Part print with two shaded views. Sizes in mm from the minimum x, y, z corner. Round coordinates to 2 decimals unless told otherwise and drop trailing zeros. Loops run counter-clockwise (first coordinate to the right, second up) from the corner with the lowest first, then second, coordinate; pieces in that order, holes last. Notation, with made-up numbers: (-13, 2) - (28, 2) arc R14 cw to (28, 26) - close; hole circle Ø5 at (42, -1.75). An arc over 180 degrees is marked (long way). One line per question, with ' | ' between items.
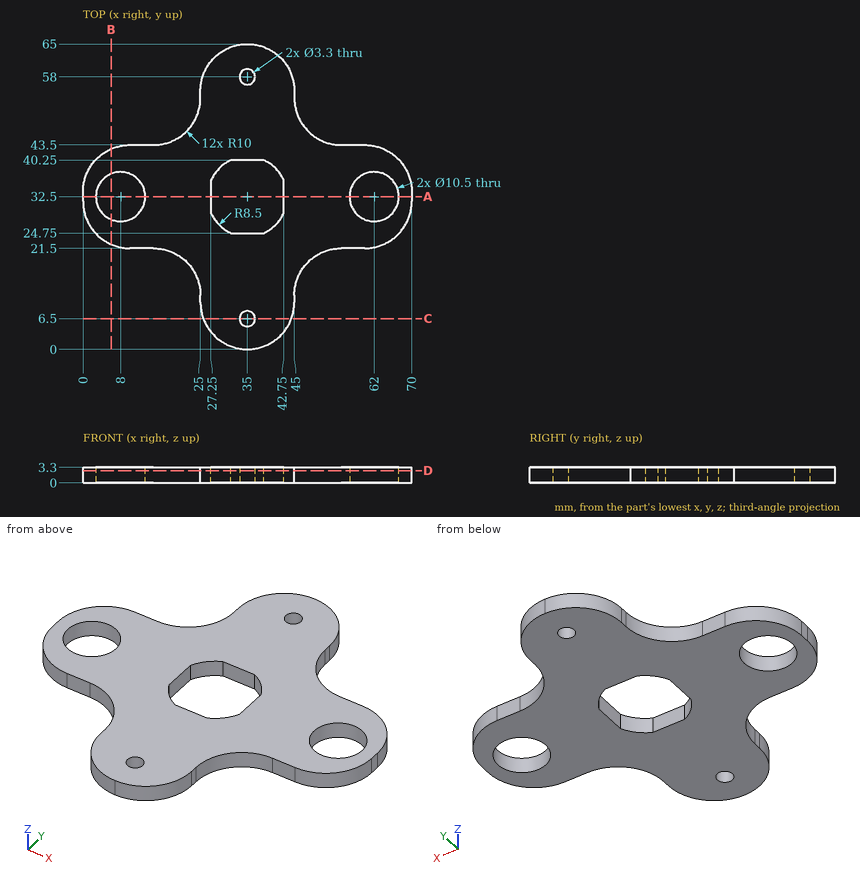
(1) Cut at C-C, the plane y = 6.5. Write the cut outline in (x, z), then the cut area to 3 significant figures.
Results found:
outline: (25.63, 0) - (33.35, 0) - (33.35, 3.3) - (25.63, 3.3) - close; (36.65, 0) - (44.37, 0) - (44.37, 3.3) - (36.65, 3.3) - close | area: 50.9 mm²
(2) Drop flat-ended pins along their axis: P1, Ø0.5, axis at y = 11, z = 1, coming from the +X side; P2, Ø1.7, axis at y = 10.5, z = 1.5, coming from the -X side; P3, Ø1.6, axis at x = 12.5, z = 2, coming from the +Y side. Give the stop position or say it passes through.
Results found:
P1: stops at x = 45 | P2: stops at x = 25 | P3: stops at y = 43.5
(3) Cut at B-B, the plane x = 6. Write the cut outline in (y, z) (3 decimals).
Results found:
outline: (22.335, 0) - (27.646, 0) - (27.646, 3.3) - (22.335, 3.3) - close; (37.354, 0) - (42.665, 0) - (42.665, 3.3) - (37.354, 3.3) - close
(4) Cut at D-D, the plane z = 2.6. State how many separate pieces and enclosed holes the cut face has, then the cut area to 3 significant figures.
Results found:
separate pieces: 1 | enclosed holes: 5 | area: 1,910 mm²
(5) Probe L1, parallel to Y at x = 35, z = 2.3; L2, parallel to X at y = 11, z = 3.15; L3, parallel to X at y = 25, z = 0.95. List the from-to ranges inside material, lowest first.
Results found:
L1: y = 0 to 4.85, 8.15 to 24.75, 40.25 to 56.35, 59.65 to 65 | L2: x = 25 to 45 | L3: x = 2.4 to 31, 39 to 67.6
(6) Cut at A-A, the plane y = 32.5. Write the cut outline in (x, z).
Results found:
outline: (0, 0) - (2.75, 0) - (2.75, 3.3) - (0, 3.3) - close; (13.25, 0) - (27.25, 0) - (27.25, 3.3) - (13.25, 3.3) - close; (42.75, 0) - (56.75, 0) - (56.75, 3.3) - (42.75, 3.3) - close; (67.25, 0) - (70, 0) - (70, 3.3) - (67.25, 3.3) - close
